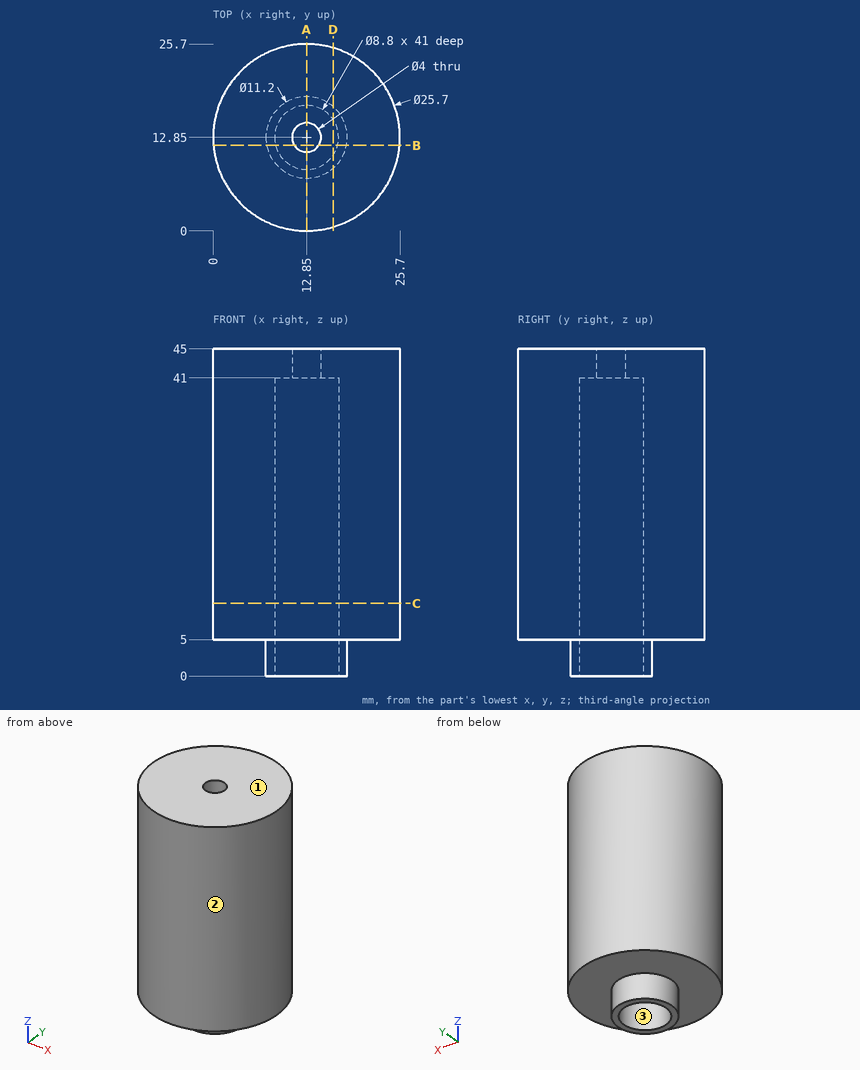
Geometry: see drawing. Coordinates: mm, zero at the bounding-box minimum. Coordinates: 2 decimals unless noted, no trailing zeros. Write each loop counter-clockwise with the first axis right and the second up, starting at its lowest first coordinate (ties: lowest second). Pieces come first, ordered by that corner, then holes. Notation, with made-up numbers: M -37,13.5 L 8,13.5 A15 ccw 8,20.5 Z; hole C 18,-28.75 d1. An arc over 180 degrees is marked long. Use CSV: the item, a comma, the result in double quotes. Start each with the question number.
1. Cut plane A-A on x = 12.85. Return the cut outline in (y, z).
2. Ray query, probe 1 along Y at (x, z) = (12.85, 42.85); probe 2 along X at (y, z) = (12.85, 14.5). Return the intervals inside material, ascending.
3. First-contact query: P1, Ø14, axis at x = 12.85, y = 12.85, coming from the +Z side; P2, Ø8, axis at x = 6, z = 17, coming from the +Y side; P3, Ø12, axis at x = 20, z = 20, coming from the -Y side; P4, Ø4.5, axis at x = 11.5, y = 13, coming from the -Z side. Flat tips, straight axial feed; report the tip coordinate or a pass-through.
4. Cut plane B-B on y = 11.75. Return the cut outline in (x, z), plus the area to 3 significant figures.
5. Cut plane D-D on x = 16.5. Return the cut outline in (y, z), plus the area to 3 significant figures.
6. Mould query, pull axis X, two halves, no side actions, for the marked faces 1, 2 and 3. Classes: pulls with the +X half, pulls with the -X half, needs draft (parallel to the pull), parting line crosses it, or undercut.
7. Cut plane C-C on z = 10. Return the cut outline in (x, y), plus the area to 3 significant figures.
Entries:
1,outline,"M 0,5 L 7.25,5 L 7.25,0 L 8.45,0 L 8.45,41 L 10.85,41 L 10.85,45 L 0,45 Z; M 14.85,41 L 17.25,41 L 17.25,0 L 18.45,0 L 18.45,5 L 25.7,5 L 25.7,45 L 14.85,45 Z"
2,probe 1,"0 to 10.85, 14.85 to 25.7"
2,probe 2,"0 to 8.45, 17.25 to 25.7"
3,P1,"z = 45"
3,P2,"y = 25.38"
3,P3,"y = 0.05"
3,P4,"z = 41"
4,outline,"M 0.05,5 L 7.36,5 L 7.36,0 L 8.59,0 L 8.59,41 L 11.18,41 L 11.18,45 L 0.05,45 Z; M 14.52,41 L 17.11,41 L 17.11,0 L 18.34,0 L 18.34,5 L 25.65,5 L 25.65,45 L 14.52,45 Z"
4,area,"716 mm²"
5,outline,"M 0.53,5 L 8.6,5 L 8.6,0 L 10.39,0 L 10.39,41 L 15.31,41 L 15.31,0 L 17.1,0 L 17.1,5 L 25.17,5 L 25.17,45 L 0.53,45 Z"
5,area,"827 mm²"
6,face 1,"needs draft"
6,face 2,"parting line crosses it"
6,face 3,"undercut"
7,outline,"C 12.85,12.85 d25.7; hole C 12.85,12.85 d8.8"
7,area,"458 mm²"
